Build history of the part. All positions in model axes, mm. A direction names the side the tool comes from. Coordinates: 2 decimals unless noted, no trailing zeros. Write each loop counter-clockwise with the first axis right and the second up, starting at its lowest first coordinate (ties: lowest second). Pieces come first, ordered by that corner, then holes.
from build123d import *

# Parameters (mm, degrees)
SKETCH1_W                                      = 12.7
SKETCH1_H                                      = 234.95
BOSS_EXTRUDE1_DEPTH                            = 90.2
SKETCH3_W                                      = 15
SKETCH3_H                                      = 15
BOSS_EXTRUDE2_DEPTH                            = 5
CSK_FOR_4_FLAT_HEAD_MACHINE_SCREW1_D           = 3.2639
CSK_FOR_4_FLAT_HEAD_MACHINE_SCREW1_DEPTH       = 5
CSK_FOR_4_FLAT_HEAD_MACHINE_SCREW1_CSINK_D     = 5.715
CSK_FOR_4_FLAT_HEAD_MACHINE_SCREW1_CSINK_ANGLE = 82
FILLET1_R                                      = 5
FILLET2_R                                      = 3


with BuildPart() as part:
    # Sketch1 → Boss-Extrude1 (new body)
    with BuildSketch(Plane(origin=(0, 0, 0), x_dir=(1, 0, 0), z_dir=(0, 1, 0))):
        Rectangle(SKETCH1_W, SKETCH1_H)
    extrude(amount=BOSS_EXTRUDE1_DEPTH)

    # Sketch3 → Boss-Extrude2 (add)
    with BuildSketch(Plane(origin=(0, 90.2, 0), x_dir=(1, 0, 0), z_dir=(0, 1, 0))):
        with Locations((-13.85, 99.975)):
            Rectangle(SKETCH3_W, SKETCH3_H)
        with Locations((-13.85, -99.975)):
            Rectangle(SKETCH3_W, SKETCH3_H)
        with Locations((-13.85, 0)):
            Rectangle(SKETCH3_W, SKETCH3_H)
    extrude(amount=-BOSS_EXTRUDE2_DEPTH)

    # CSK for #4 Flat Head Machine Screw1
    with Locations(Plane.XZ.offset(-85.2)):
        with Locations((-13.85, 99.975), (-13.85, 0), (-13.85, -99.975)):
            CounterSinkHole(CSK_FOR_4_FLAT_HEAD_MACHINE_SCREW1_D / 2, CSK_FOR_4_FLAT_HEAD_MACHINE_SCREW1_CSINK_D / 2, depth=CSK_FOR_4_FLAT_HEAD_MACHINE_SCREW1_DEPTH, counter_sink_angle=CSK_FOR_4_FLAT_HEAD_MACHINE_SCREW1_CSINK_ANGLE)

    # Fillet1
    fillet1_edges = [part.edges().sort_by_distance(p)[0] for p in [
        (-6.35, 87.7, -107.475),
        (-6.35, 87.7, -92.475),
        (-21.35, 87.7, -92.475),
        (-21.35, 87.7, -107.475),
        (-6.35, 87.7, 92.475),
        (-6.35, 87.7, 107.475),
        (-21.35, 87.7, 107.475),
        (-21.35, 87.7, 92.475),
        (-21.35, 87.7, 7.5),
        (-21.35, 87.7, -7.5),
        (-6.35, 87.7, -7.5),
        (-6.35, 87.7, 7.5),
    ]]
    fillet(fillet1_edges, radius=FILLET1_R)

    # Fillet2
    fillet2_edges = [part.edges().sort_by_distance(p)[0] for p in [
        (-6.35, 85.2, -99.975),
        (-6.35, 85.2, 99.975),
        (-6.35, 85.2, 0),
    ]]
    fillet(fillet2_edges, radius=FILLET2_R)


solid = part.part
(1) Slice it at A-A, the plane y = 60. List the corners of the cut face in (x, z) (3 decimals).
(2) Flat gauge pins, fed straight in: P1, Ø5.5, axis at x = -14, y = 86.5, coming from the -Z side; P2, Ø1.5, axis at x = -14, y = 89, coming from the +Z side (3 decimals); P3, Ø6, axis at x = -12, y = 81, coming from the -Z side; P4, Ø5.5, axis at x = -12.5, y = 87.5, coming from the -Z side. Where does each tip first touch, or does it go through?
(3) Probe L1, parallel to Z at x = -13.85, y = 88.35 (3 decimals); L2, parallel to X at y = 87.4, z = 0; L3, parallel to X at y = 54, z = 54.5. List the from-to ranges inside material, lowest first.
(4) 3-axis set-ups, long thin cutter, end or side, ignore diameter. For faces 1 (the cylindrical face through (-7.776, 87.033, 90.971)), 2 (the flat face through (-17, 85.2, 100)), 3 (the cylindrical face through (-19.924, 87.665, -105.971)): which of +Z, -Z, +X, -X, +Y, -Y reach the whole face in a straight line?
(5) Two-plate mould, pull along Z, no slides. Class faces 4 (the cylindrical face through (-7.78, 87.03, -9)), 5 (the flat face through (0, 44, 117.475)), 6 (the cylindrical face through (-7.776, 87.033, -90.971)), 7 (the flat face through (-21.35, 88, 100)): pulls with the +Z half, pulls with the -Z half, needs draft (parallel to the pull), parting line crosses it, or undercut.
(6) Slice it at B-B, the plane z = 65.5. List the corners of the cut face in (x, y), and give its area (3 significant figures).
Results:
1. outline: (-6.35, -117.475) - (6.35, -117.475) - (6.35, 117.475) - (-6.35, 117.475) - close
2. P1: stops at z = -107.48
2. P2: stops at z = 107.475
2. P3: passes through
2. P4: stops at z = -107.74
3. L1: z = -107.475 to -101.607, -98.343 to -92.475, -7.5 to -1.632, 1.632 to 7.5, 92.475 to 98.343, 101.607 to 107.475
3. L2: x = -21.35 to -15.48, -12.22 to 6.35
3. L3: x = -6.35 to 6.35
4. face 1: -X, +Y, -Y
4. face 2: +Z, -Z, -X, -Y
4. face 3: -Z, -X, +Y, -Y
5. face 4: undercut
5. face 5: pulls with the +Z half
5. face 6: undercut
5. face 7: needs draft
6. outline: (-6.35, 0) - (6.35, 0) - (6.35, 90.2) - (-6.35, 90.2) - close
6. area: 1,150 mm2
